Could you check a few things on this model? Use its own coordinates, in mm. Face numbers are marked on the shaded views. A direction names the side the tool comes from. Coordinates: 2 decimals unless noted, no trailing zeros. Write each loop counter-clockwise with the first axis right and the second up, starting at its lowest first coordinate (ties: lowest second). Pieces come first, ordered by that corner, then holes. Notation, with made-up numbers: (-6.75, 13.25) - (6.25, 13.25) arc R25 cw to (6.25, 38.25) - close; hole circle Ø3 at (-5.5, 13.5). An arc over 180 degrees is marked (long way). Answer as a JSON object with one key per item and string values. Group by question number.
1) If we section it at A-A (x = 25.4): Write out the boundary of the cut face in (y, z) (3 decimals), plus the area to 3 significant figures.
2) Will these pins go through, and if not, where does the flat tip stop? pin 1 Ø2 at (y, z) = (-39.5, 6.5) entering from -X; pin 2 Ø15 at (x, y) = (234.95, -88.9) entering from +Z; pin 3 Ø3 at (x, z) = (122, 18) entering from -Y.
3) On a 3-axis mill with a long thin cutter (end or side, diameter ignored), from which of +Z, -Z, +X, -X, +Y, -Y can I reach the whole of each face in a straight line? I mean the marked faces 1 and 2. Say none if no direction works.
4) If we section it at D-D (y = -33): Write out the boundary of the cut face in (x, z), plus the area to 3 significant figures.
5) If we section it at C-C (z = 8.25): Write out the boundary of the cut face in (x, y) (3 decimals), plus the area to 3 significant figures.
6) If we section it at B-B (y = 19.05): Write out the boundary of the cut face in (x, z) (3 decimals).
7) Please list where these lines run through material, in increasing order: line 1 along Y through (x, z) = (234.95, 18.25) (3 decimals); line 2 along Y through (x, z) = (25.4, 18.25) (3 decimals); line 3 along Y through (x, z) = (55.5, 13.5).
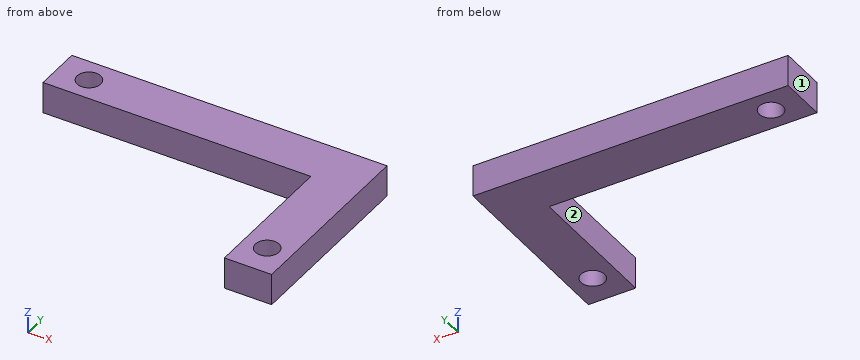
```python
from build123d import *

# Parameters (mm, degrees)
SKETCH1_W           = 254
SKETCH1_H           = 38.1
SKETCH1_W_2         = 38.1
SKETCH1_H_2         = 114.3
BOSS_EXTRUDE1_DEPTH = 25.4
SKETCH2_R           = 9.525
CUT_EXTRUDE1_DEPTH  = 280.688487428
SKETCH3_R           = 9.525
CUT_EXTRUDE2_DEPTH  = 280.688487428


with BuildPart() as part:
    # Sketch1 → Boss-Extrude1 (new body)
    with BuildSketch(Plane.XY):
        with Locations((127, 19.05)):
            Rectangle(SKETCH1_W, SKETCH1_H)
        with Locations((234.95, -57.15)):
            Rectangle(SKETCH1_W_2, SKETCH1_H_2)
    extrude(amount=BOSS_EXTRUDE1_DEPTH)

    # Sketch2 → Cut-Extrude1 (cut, through all)
    with BuildSketch(Plane.XY.offset(25.4)):
        with Locations((25.4, 19.05)):
            Circle(SKETCH2_R)
    extrude(amount=-CUT_EXTRUDE1_DEPTH, mode=Mode.SUBTRACT)

    # Sketch3 → Cut-Extrude2 (cut, through all)
    with BuildSketch(Plane.XY.offset(25.4)):
        with Locations((234.95, -88.9)):
            Circle(SKETCH3_R)
    extrude(amount=-CUT_EXTRUDE2_DEPTH, mode=Mode.SUBTRACT)


solid = part.part
```
Here are the results:
{
 "1": {"outline": "(0, 0) - (9.525, 0) - (9.525, 25.4) - (0, 25.4) - close; (28.575, 0) - (38.1, 0) - (38.1, 25.4) - (28.575, 25.4) - close", "area": "484 mm²"},
 "2": {"pin 1": "stops at x = 215.9", "pin 2": "passes through", "pin 3": "stops at y = 0"},
 "3": {"face 1": "+Z, -Z, -X, +Y, -Y", "face 2": "+Z, -Z, -X, -Y"},
 "4": {"outline": "(215.9, 0) - (254, 0) - (254, 25.4) - (215.9, 25.4) - close", "area": "968 mm²"},
 "5": {"outline": "(0, 0) - (215.9, 0) - (215.9, -114.3) - (254, -114.3) - (254, 38.1) - (0, 38.1) - close; hole circle Ø19.05 at (25.4, 19.05); hole circle Ø19.05 at (234.95, -88.9)", "area": "13,500 mm²"},
 "6": {"outline": "(0, 0) - (15.875, 0) - (15.875, 25.4) - (0, 25.4) - close; (34.925, 0) - (254, 0) - (254, 25.4) - (34.925, 25.4) - close"},
 "7": {"line 1": "y = -114.3 to -98.425, -79.375 to 38.1", "line 2": "y = 0 to 9.525, 28.575 to 38.1", "line 3": "y = 0 to 38.1"}
}
